```python
from build123d import *

# Parameters (mm, degrees)
F0_W     = 40
F0_H     = 36
F1_DEPTH = 50
F2_R     = 5
F3_DEPTH = 45
F4_W     = 40
F4_H     = 6.8
F5_DEPTH = 45
F6_R     = 19.99999
F7_R     = 4
F8_DEPTH = 50


# Not quite as in the source:
# - a fillet or chamfer is up to 0.001 mm smaller than in the source, because OpenCascade refuses the exact size


with BuildPart() as f1:
    # F0 (on Top) → F1 (new body)
    with BuildSketch(Plane.XY):
        Rectangle(F0_W, F0_H)
    extrude(amount=F1_DEPTH)

    # F2 (on face) → F3 (cut)
    with BuildSketch(Plane.YZ.offset(20)):
        with Locations((0, 42)):
            Circle(F2_R)
        with Locations((0, 8)):
            Circle(F2_R)
    extrude(amount=-F3_DEPTH, mode=Mode.SUBTRACT)

    # F4 (on face) → F5 (join)
    with BuildSketch(Plane.XY.offset(50)):
        with Locations((0, -14.6)):
            Rectangle(F4_W, F4_H)
        with Locations((0, 14.6)):
            Rectangle(F4_W, F4_H)
    extrude(amount=F5_DEPTH)

    # F6 (radius 20 in the source; OpenCascade refuses exactly that, so slightly less here)
    f6_edges = [f1.edges().sort_by_distance(p)[0] for p in [
        (20, 14.6, 95),
        (20, -14.6, 95),
        (-20, 14.6, 95),
        (-20, -14.6, 95),
    ]]
    fillet(f6_edges, radius=F6_R)

    # F7 (on face) → F8 (cut)
    with BuildSketch(Plane(origin=(0, 18, 0), x_dir=(-1, 0, 0), z_dir=(0, 1, 0))):
        with Locations((0, 79)):
            Circle(F7_R)
    extrude(amount=-F8_DEPTH, mode=Mode.SUBTRACT)


solid = f1.part
```
Geometry check sheet. Reference: the model listing, model coordinates, mm. A direction names the side the tool comes from. Give positions to 0.01 mm unless a question says otherwise; leave off trailing zeros. Loops run counter-clockwise (first coordinate to the right, second up) from the corner with the lowest first, then second, coordinate; pieces in that order, holes last. Notation, with made-up numbers: M 2,-10 L 45,-10 A34 ccw 45,29 Z; hole C 89.25,-26 d8. An arc over 180 degrees is marked long. Write item = value, one per line. Start each with the question number.
1. Go/stop test with flat-tipped pins: P1, Ø6.5, axis at x = 0, z = 79, coming from the -Y side; P2, Ø1.5, axis at x = -3.5, y = 11, coming from the -Z side. Record where each tip stops, or that it passes through.
2. Section check C-C, the plane z = 8. Enter the section's corners in (x, y).
3. Tool access check on faces 4 (the face through (0, -11.2, 72)), 5 (the face through (0.28, -0.651, 46.957)). Record the directions out of +Z, -Z, +X, -X, +Y, -Y that give a thin tool (end or side, any length) a straight path to the whole face; none if there is none.
4. Thickness scan on probe 1 along Z at (x, y) = (6, 0); probe 2 along Y at (x, z) = (16.5, 86); probe 3 along Z at (x, y) = (0, -15.25). Record the ranges inside material, lowest first.
5. Draft check along Y on faces 1 (the face through (-20, 0, 29)), 2 (the face through (0, 18, 47)), 3 (the face through (0, 11.2, 72)). Enter one of: +Y half, -Y half, draft (parallel to the pull), parting line (faces both ways), or undercut.
6. Section check A-A, the plane y = -3. Enter the section's corners in (x, z).
7. Section check B-B, the plane x = -12. Enter the section's corners in (y, z), plus the area to 3 significant figures.
8. Section check D-D, the plane z = 79. Enter the section's corners in (x, y).
Values follow:
q1.P1 = through
q1.P2 = 0
q2.outline = M -20,-18 L 20,-18 L 20,-5 L -20,-5 Z; M -20,5 L 20,5 L 20,18 L -20,18 Z
q3.face_4 = +Z, +X, -X
q3.face_5 = +X, -X
q4.probe_1 = 0 to 3, 13 to 37, 47 to 50
q4.probe_2 = -18 to -11.2, 11.2 to 18
q4.probe_3 = 0 to 75, 83 to 95
q5.face_1 = draft
q5.face_2 = +Y half
q5.face_3 = undercut
q6.outline = M -20,0 L 20,0 L 20,4 L -20,4 Z; M -20,12 L 20,12 L 20,38 L -20,38 Z; M -20,46 L 20,46 L 20,50 L -20,50 Z
q7.outline = M -18,0 L 18,0 L 18,91 L 11.2,91 L 11.2,50 L -11.2,50 L -11.2,91 L -18,91 Z; hole C 0,8 d10; hole C 0,42 d10
q7.area = 2,200 mm^2
q8.outline = M -19.6,-18 L -4,-18 L -4,-11.2 L -19.6,-11.2 Z; M -19.6,11.2 L -4,11.2 L -4,18 L -19.6,18 Z; M 4,-18 L 19.6,-18 L 19.6,-11.2 L 4,-11.2 Z; M 4,11.2 L 19.6,11.2 L 19.6,18 L 4,18 Z
